Verification items for the finished model (mm, model axes). A direction names the side the tool comes from. Give positions to 0.01 mm unless a question says otherwise; leave off trailing zeros. Write each loop counter-clockwise with the first axis right and the second up, starting at its lowest first coordinate (ties: lowest second). Pieces come first, ordered by that corner, then holes.
from build123d import *

# Parameters (mm, degrees)
BOX017_W        = 17.2
BOX017_H        = 4.3
BOX017_DEPTH    = 1
BOX016_W        = 16.2
BOX016_H        = 3.3
BOX016_DEPTH    = 8
CHAMFER_SIZE    = 0.9
CHAMFER001_SIZE = 0.9


with BuildPart() as tapa_puerta001:
    # Box017 → Box017 (new body)
    with BuildSketch(Plane(origin=(80.5, -27.5, 22.8), x_dir=(1, 0, 0), z_dir=(0, 0, 1))):
        with Locations((8.6, 2.15)):
            Rectangle(BOX017_W, BOX017_H)
    extrude(amount=BOX017_DEPTH)


with BuildPart() as tapa_puerta:
    # Box016 → Box016 (new body)
    with BuildSketch(Plane(origin=(81, -27, 14.8), x_dir=(1, 0, 0), z_dir=(0, 0, 1))):
        with Locations((8.1, 1.65)):
            Rectangle(BOX016_W, BOX016_H)
    extrude(amount=BOX016_DEPTH)

    # Fusion006: union tapa_puerta001
    add(tapa_puerta001.part)

    # Chamfer
    chamfer_edges = [tapa_puerta.edges().sort_by_distance(p)[0] for p in [
        (89.1, -23.2, 23.8),
    ]]
    chamfer(chamfer_edges, length=CHAMFER_SIZE)

    # Chamfer001
    chamfer001_edges = [tapa_puerta.edges().sort_by_distance(p)[0] for p in [
        (80.5, -25.8, 23.8),
        (89.1, -27.5, 23.8),
        (97.7, -25.8, 23.8),
    ]]
    chamfer(chamfer001_edges, length=CHAMFER001_SIZE)


with BuildPart() as tapa_puerta_1:
    # Chamfer001 placement: moved
    add(tapa_puerta.part.moved(Location((0, 0, 2))))


solid = tapa_puerta_1.part
Item 1: Sectioned sample at C-C on z = 19.5. Record the cut outline in (x, y), then the cut area to 3 significant figures.
Answer key:
outline: (81, -27) - (97.2, -27) - (97.2, -23.7) - (81, -23.7) - close
area: 53.5 mm2
Item 2: Sectioned sample at B-B on x = 83.5. Record the cut outline in (y, z), then the cut area to 3 significant figures.
Answer key:
outline: (-27.5, 24.8) - (-27, 24.8) - (-27, 16.8) - (-23.7, 16.8) - (-23.7, 24.8) - (-23.2, 24.8) - (-23.2, 24.9) - (-24.1, 25.8) - (-26.6, 25.8) - (-27.5, 24.9) - close
area: 29.9 mm2
Item 3: Scan lines: line 1 along Y through (x, z) = (83, 22); line 2 along X through (y, z) = (-25.7, 21); line 3 along Z through (x, y) = (89.75, -26.8). Record each from-to range of solid material in increasing order.
Answer key:
line 1: y = -27 to -23.7
line 2: x = 81 to 97.2
line 3: z = 16.8 to 25.6
Item 4: Set-up check for faces 1 (the face through (97.2, -25, 21)), 2 (the face through (81, -25, 21)), 3 (the face through (89, -23.7, 21)): record each of +Z, -Z, +X, -X, +Y, -Y from which the full face is reachable in a straight line by a thin tool's end or side.
Answer key:
face 1: -Z, +X, +Y, -Y
face 2: -Z, -X, +Y, -Y
face 3: -Z, +X, -X, +Y
Item 5: Sectioned sample at A-A on y = -26.8. Record the cut outline in (x, z), then the cut area to 3 significant figures.
Answer key:
outline: (80.5, 24.8) - (81, 24.8) - (81, 16.8) - (97.2, 16.8) - (97.2, 24.8) - (97.7, 24.8) - (97.7, 24.9) - (97, 25.6) - (81.2, 25.6) - (80.5, 24.9) - close
area: 143 mm2
Item 6: Depth check by flat-ended pin: pin 1 (4 mm diameter, centred on x = 85.5, z = 20.5, fed in from -Y); pin 2 (2.5 mm diameter, centred on x = 91, z = 20.5, fed in from +Y); pin 3 (1.6 mm diameter, centred on y = -25.5, z = 20, fed in from +X). Enter the tip coordinate at first touch or a pass-through.
Answer key:
pin 1: stops at y = -27
pin 2: stops at y = -23.7
pin 3: stops at x = 97.2
